Part model, mm, in its own coordinate system. Face numbers are marked on the shaded views. Round coordinates to 2 decimals unless told otherwise and drop trailing zeros. Order: outer loops, then holes, each group sorted by start corner. A loop starts at its lowest first (then second) coordinate and runs counter-clockwise, first axis right, second up. Notation, with made-up numbers: (75.5, -23.75) - (90.5, -23.75) arc R35 ccw to (90.5, 11.25) - close; hole circle Ø1 at (12, 26.25). An arc over 180 degrees is marked (long way). Return JSON: item names as keys, results as strings. Group by question number.
Item 1: Two-plate mould, pull along Z, no slides. Class the marked faces 1, 2 and 3: released by +Z, released by -Z, zero draft, split by the parting line, or undercut.
Item 2: Drop flat-ended pins along their axis: pin 1 (4.5 mm diameter, centred on x = -21.5, y = 10.5, fed in from +Z); pin 2 (1.5 mm diameter, centred on x = -3.5, y = 9.5, fed in from +Z); pin 3 (2 mm diameter, centred on y = 11, z = 28.5, fed in from +X); pin 4 (13 mm diameter, centred on x = -6, z = 2.5, fed in from +Y). Give the stop position or say it passes through.
Item 3: Saw through at A-A on z = 15. List the corners of the cut face in (x, y).
Item 4: Saw through at B-B on x = -31. List the corners of the cut face in (y, z), and give its area (3 significant figures).
Item 5: Saw through at C-C on y = 2. List the corners of the cut face in (x, z).
Item 6: Probe probe 1 along X at (y, z) = (2, -5); probe 2 along X at (y, z) = (1.7, 40); probe 3 along Z at (x, y) = (-31, 1.5). List the from-to ranges inside material, lowest first.
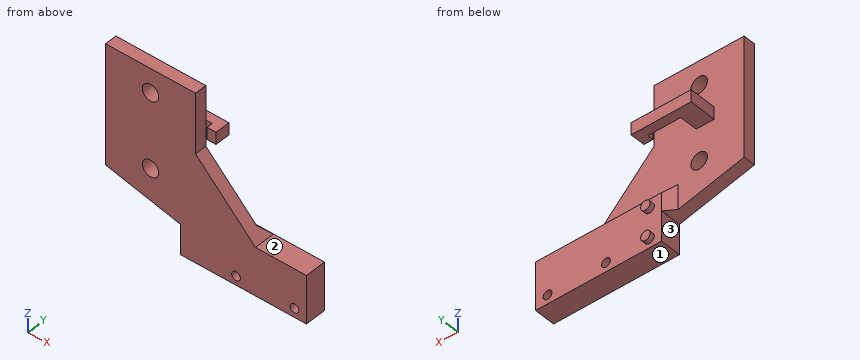
```python
from build123d import *

# Parameters (mm, degrees)
SKETCH1_W           = 42
SKETCH1_H           = 16
BOSS_EXTRUDE1_DEPTH = 7
SKETCH2_R           = 1.6
BOSS_EXTRUDE2_DEPTH = 1.6
CUT_EXTRUDE1_REACH  = 26.062
SKETCH3_R           = 1.45
BOSS_EXTRUDE6_DEPTH = 4
CUT_EXTRUDE2_REACH  = 69.037
SKETCH8_R           = 2.75
BOSS_EXTRUDE7_DEPTH = 2
CHAMFER2_SIZE       = 3


with BuildPart() as part:
    # Sketch1 → Boss-Extrude1 (new body)
    with BuildSketch(Plane(origin=(0, 0, 0), x_dir=(1, 0, 0), z_dir=(0, 1, 0))):
        Rectangle(SKETCH1_W, SKETCH1_H)
    extrude(amount=BOSS_EXTRUDE1_DEPTH)

    # Sketch2 → Boss-Extrude2 (add)
    with BuildSketch(Plane(origin=(0, 7, 0), x_dir=(1, 0, 0), z_dir=(0, 1, 0))):
        with Locations(Location((-17, 5, 0), (0, 0, 270))):
            Circle(SKETCH2_R)
        with Locations(Location((-17, -5, 0), (0, 0, 270))):
            Circle(SKETCH2_R)
    extrude(amount=BOSS_EXTRUDE2_DEPTH)

    # Sketch3 → Cut-Extrude1 (cut, up to next)
    with BuildSketch(Plane(origin=(0, 0, 0), x_dir=(1, 0, 0), z_dir=(0, 1, 0)), mode=Mode.PRIVATE) as cut_extrude1_sk1:
        with Locations(Location((-2.5, 5, 0), (0, 0, 270))):
            Circle(SKETCH3_R)
    cut_extrude1_tool1 = extrude(cut_extrude1_sk1.sketch, amount=CUT_EXTRUDE1_REACH, mode=Mode.PRIVATE) & part.part
    # Sketch3 → Cut-Extrude1 (cut, up to next)
    with BuildSketch(Plane(origin=(0, 0, 0), x_dir=(1, 0, 0), z_dir=(0, 1, 0)), mode=Mode.PRIVATE) as cut_extrude1_sk2:
        with Locations(Location((17, 5, 0), (0, 0, 270))):
            Circle(SKETCH3_R)
    cut_extrude1_tool2 = extrude(cut_extrude1_sk2.sketch, amount=CUT_EXTRUDE1_REACH, mode=Mode.PRIVATE) & part.part
    add(cut_extrude1_tool1.solids().sort_by_distance((-2.5, 0, -5))[0], mode=Mode.SUBTRACT)
    add(cut_extrude1_tool2.solids().sort_by_distance((17, 0, -5))[0], mode=Mode.SUBTRACT)

    # Sketch7 → Boss-Extrude6 (add)
    with BuildSketch(Plane(origin=(0, 0, 0), x_dir=(1, 0, 0), z_dir=(0, 1, 0))):
        Polygon((-21, -2), (-46, -8), (-46, -48), (-16, -48), (-16, -28), (4, -8), (-21, -8), align=None)
    extrude(amount=BOSS_EXTRUDE6_DEPTH)

    # Sketch8 → Cut-Extrude2 (cut, up to next)
    with BuildSketch(Plane(origin=(0, 0, 0), x_dir=(1, 0, 0), z_dir=(0, 1, 0)), mode=Mode.PRIVATE) as cut_extrude2_sk1:
        with Locations(Location((-31, -40, 0), (0, 0, 90))):
            Circle(SKETCH8_R)
    cut_extrude2_tool1 = extrude(cut_extrude2_sk1.sketch, amount=CUT_EXTRUDE2_REACH, mode=Mode.PRIVATE) & part.part
    # Sketch8 → Cut-Extrude2 (cut, up to next)
    with BuildSketch(Plane(origin=(0, 0, 0), x_dir=(1, 0, 0), z_dir=(0, 1, 0)), mode=Mode.PRIVATE) as cut_extrude2_sk2:
        with Locations(Location((-31, -15, 0), (0, 0, 90))):
            Circle(SKETCH8_R)
    cut_extrude2_tool2 = extrude(cut_extrude2_sk2.sketch, amount=CUT_EXTRUDE2_REACH, mode=Mode.PRIVATE) & part.part
    add(cut_extrude2_tool1.solids().sort_by_distance((-31, 0, 40))[0], mode=Mode.SUBTRACT)
    add(cut_extrude2_tool2.solids().sort_by_distance((-31, 0, 15))[0], mode=Mode.SUBTRACT)

    # Sketch9 → Boss-Extrude7 (add, symmetric)
    with BuildSketch(Plane.XY.offset(28)):
        Polygon((-36, 4), (-36, 13), (-16, 13), (-16, 8), (-19, 8), (-19, 10), (-30, 10), (-30, 4), align=None)
    extrude(amount=BOSS_EXTRUDE7_DEPTH, both=True)

    # Chamfer2
    chamfer2_edges = [part.edges().sort_by_distance(p)[0] for p in [
        (-21, 4, 5),
        (-8.5, 4, 8),
    ]]
    chamfer(chamfer2_edges, length=CHAMFER2_SIZE - 0.0001)  # a hair under: the kernel refuses the full size


solid = part.part
```
Filled in:
{
 "1": {"face 1": "released by -Z", "face 2": "released by +Z", "face 3": "zero draft"},
 "2": {"pin 1": "stops at z = 30", "pin 2": "passes through", "pin 3": "stops at x = -16", "pin 4": "stops at y = 7"},
 "3": {"outline": "(-46, 0) - (-33.75, 0) - (-33.75, 4) - (-46, 4) - close; (-28.25, 0) - (-3, 0) - (-3, 4) - (-28.25, 4) - close"},
 "4": {"outline": "(0, 4.4) - (4, 4.4) - (4, 12.25) - (0, 12.25) - close; (0, 17.75) - (4, 17.75) - (4, 26) - (13, 26) - (13, 30) - (4, 30) - (4, 37.25) - (0, 37.25) - close; (0, 42.75) - (4, 42.75) - (4, 48) - (0, 48) - close", "area": "166 mm^2"},
 "5": {"outline": "(-46, 8) - (-21, 2) - (-21, -8) - (21, -8) - (21, 8) - (4, 8) - (-16, 28) - (-16, 48) - (-46, 48) - close; hole circle Ø5.5 at (-31, 15); hole circle Ø5.5 at (-31, 40); hole circle Ø2.9 at (-2.5, -5); hole circle Ø2.9 at (17, -5)"},
 "6": {"probe 1": "x = -21 to -3.95, -1.05 to 15.55, 18.45 to 21", "probe 2": "x = -46 to -33.75, -28.25 to -16", "probe 3": "z = 4.4 to 12.25, 17.75 to 37.25, 42.75 to 48"}
}
